from build123d import *

# Parameters (mm, degrees)
F0_R     = 0.4318
F1_DEPTH = 1.27


with BuildPart() as f1:
    # F0 (on Top) → F1 (new body)
    with BuildSketch(Plane.XY):
        with BuildLine():
            Line((12.65347, -2.153963), (4.316134, 2.261672))
            Line((4.316134, 2.261672), (4.327364, 12.763659))
            Line((4.327364, 12.763659), (4.156866, 12.998858))
            ThreePointArc((4.156866, 12.998858), (2.963087, 14.80923), (1.900066, 12.919114))
            Line((1.900066, 12.919114), (1.711051, 12.659542))
            Line((1.711051, 12.659542), (1.699981, 2.307537))
            Line((1.699981, 2.307537), (-5.691423, -1.091549))
            Line((-5.691423, -1.091549), (-5.691423, -2.478054))
            Line((-5.691423, -2.478054), (-5.310308, -2.303015))
            Line((-5.310308, -2.303015), (3.007935, 1.517402))
            Line((3.007935, 1.517402), (11.38347, -2.918464))
            Line((11.38347, -2.918464), (11.38347, -3.767079))
            Line((11.38347, -3.767079), (11.38347, -4.793607))
            Line((11.38347, -4.793607), (11.383473, -10.512839))
            Line((11.383473, -10.512839), (11.383474, -11.539368))
            Line((11.383474, -11.539368), (11.383474, -12.419249))
            Line((11.383474, -12.419249), (3.128473, -17.185279))
            Line((3.128473, -17.185279), (2.03357, -16.553137))
            Line((2.03357, -16.553137), (1.14457, -16.039872))
            Line((1.14457, -16.039872), (-3.808432, -13.180257))
            Line((-3.808432, -13.180257), (-5.529587, -12.419254))
            Line((-5.529587, -12.419254), (-5.691423, -3.510934))
            Line((-5.691423, -3.510934), (-6.522282, -3.510934))
            Line((-6.522282, -3.510934), (-6.580308, -3.439569))
            Line((-6.580308, -3.439569), (-6.396528, -9.918688))
            Line((-6.396528, -9.918688), (-16.026936, -16.915588))
            Line((-16.026936, -16.915588), (-16.107216, -17.162667))
            ThreePointArc((-16.107216, -17.162667), (-16.212667, -19.229532), (-14.225404, -18.651748))
            Line((-14.225404, -18.651748), (-13.96561, -18.651748))
            Line((-13.96561, -18.651748), (-6.396528, -13.152489))
            Line((-6.396528, -13.152489), (1.39857, -17.652989))
            Line((1.39857, -17.652989), (1.39857, -18.651748))
            Line((1.39857, -18.651748), (1.39857, -21.191748))
            Line((1.39857, -21.191748), (2.28757, -21.191748))
            Line((2.28757, -21.191748), (2.28757, -20.055981))
            Line((2.28757, -20.055981), (3.207054, -21.186821))
            Line((3.207054, -21.186821), (4.037913, -21.191748))
            Line((4.037913, -21.191748), (4.037913, -18.646821))
            Line((4.037913, -18.646821), (4.037913, -18.126682))
            Line((4.037913, -18.126682), (12.653472, -13.152485))
            Line((12.653472, -13.152485), (20.12443, -15.416135))
            Line((20.12443, -15.416135), (20.12443, -16.178135))
            Line((20.12443, -16.178135), (20.12443, -18.718135))
            Line((20.12443, -18.718135), (21.140028, -18.718135))
            Line((21.140028, -18.718135), (21.140028, -17.745525))
            Line((21.140028, -17.745525), (21.809838, -18.718135))
            Line((21.809838, -18.718135), (22.763277, -18.718135))
            Line((22.763277, -18.718135), (22.763277, -16.215688))
            Line((22.763277, -16.215688), (29.330721, -7.616372))
            Line((29.330721, -7.616372), (23.89467, 0.487487))
            Line((23.89467, 0.487487), (23.89467, 0.851521))
            Line((23.89467, 0.851521), (23.89467, 3.027487))
            Line((23.89467, 3.027487), (23.00567, 3.027487))
            Line((23.00567, 3.027487), (23.00567, 2.007953))
            Line((23.00567, 2.007953), (22.273508, 3.027487))
            Line((22.273508, 3.027487), (21.384508, 3.027487))
            Line((21.384508, 3.027487), (21.384508, 1.132124))
            Line((21.384508, 1.132124), (12.65347, -2.153963))
        make_face()
        with Locations((-15.424598, -18.233617)):
            Circle(F0_R, mode=Mode.SUBTRACT)
        with BuildLine():
            Line((-14.7405, -17.163612), (-6.396528, -11.017552))
            Line((-6.396528, -11.017552), (-6.396528, -12.053624))
            Line((-6.396528, -12.053624), (-14.247226, -17.75749))
            ThreePointArc((-14.247226, -17.75749), (-14.447644, -17.422161), (-14.7405, -17.163612))
        make_face(mode=Mode.SUBTRACT)
        Polygon((2.28757, -18.166253), (3.128473, -18.651748), (3.128473, -19.879702), (2.28757, -18.646821), align=None, mode=Mode.SUBTRACT)
        Polygon((21.874277, -17.244328), (21.140028, -16.178135), (21.140028, -15.723854), (21.874277, -15.946327), (21.874277, -16.178135), align=None, mode=Mode.SUBTRACT)
        Polygon((12.653474, -11.882485), (12.65347, -3.510934), (13.49167, -3.195462), (13.49167, -12.154831), align=None, mode=Mode.SUBTRACT)
        Polygon((27.564501, -6.689476), (28.079566, -7.398402), (22.323207, -15.02437), (21.47986, -14.75035), align=None, mode=Mode.SUBTRACT)
        Polygon((23.00567, 0.487487), (23.00567, -0.414785), (27.016591, -5.935343), (20.685605, -14.492281), (14.38067, -12.443685), (14.38067, -2.860871), (22.259525, 0.104481), (22.259525, 0.487487), (22.259525, 1.524642), align=None, mode=Mode.SUBTRACT)
        with BuildLine():
            Line((3.392922, 12.32978), (3.427035, 2.169838))
            Line((3.427035, 2.169838), (2.588835, 2.169838))
            Line((2.588835, 2.169838), (2.599707, 12.33742))
            ThreePointArc((2.599707, 12.33742), (2.995703, 12.270081), (3.392922, 12.32978))
        make_face(mode=Mode.SUBTRACT)
        with Locations((3.007935, 13.540022)):
            Circle(F0_R, mode=Mode.SUBTRACT)
        Polygon((-8.330766, -0.970934), (-7.652898, -0.970934), (-16.021372, 3.877039), (-16.676927, 2.740892), (-8.330766, -2.189404), align=None)
        Polygon((-5.691423, -2.478054), (-5.691423, -1.091549), (-5.691423, -0.970934), (-6.580423, -0.970934), (-6.580423, -2.198888), (-7.441766, -0.970934), (-7.652898, -0.970934), (-8.330766, -0.970934), (-8.330766, -2.189404), (-8.330766, -3.510934), (-7.441766, -3.510934), (-7.441766, -2.380094), (-6.580308, -3.439569), (-6.522282, -3.510934), (-5.691423, -3.510934), align=None)
        Polygon((24.531044, 11.272838), (23.00567, 3.027487), (23.89467, 3.027487), (23.89467, 0.851521), (25.779854, 11.04181), align=None)
    extrude(amount=F1_DEPTH)


solid = f1.part
Could you check a few things on this model? Use its own coordinates, in mm. A direction names the side the tool comes from. Give positions to 0.01 mm unless a question says otherwise; leave off trailing zeros. Write each loop counter-clockwise with the first axis right and the second up, starting at its lowest first coordinate (ties: lowest second). Pieces come first, ordered by that corner, then holes. Notation, with made-up numbers: (-16, 51) -> (-7, 51) arc R25 cw to (-7, 75) -> close; hole circle Ø10 at (75, 88.5). An arc over 180 degrees is marked (long way). Write each question's results on one line, items separated by ' | '. Start each with the question number.
Q1. I need wall thicknesses on probe 1 along Y at (x, z) = (-13, 0.1); probe 2 along X at (y, z) = (-6.5, 0.2); probe 3 along X at (y, z) = (-4, 0.45). Which ranges of each line are inside material? Lowest first, please.
Q2. I'm going to push flat-ended pins straight in: pin 1 Ø0.6 at (y, z) = (-7.5, 1) entering from -X; pin 2 Ø0.6 at (y, z) = (-2.5, 0.5) entering from +X; pin 3 Ø0.5 at (y, z) = (-11.5, 0.5) entering from -X. Where does each tip first touch, or does it pass through?
Q3. Suppose I cut it at C-C, the plane x = -12. List the corners of the cut face in (y, z) for me (3 decimals), and give its area (3 significant figures).
Q4. Which directions (+Z, -Z, +X, -X, +Y, -Y) give clear straight access to the entire face, cutting with the end or side of a thin tool? Please do faces 1 (the face through (20.124, -17, 1)), 2 (the face through (-6, -0.971, 1)), 3 (the face through (-8, -3.511, 1)), 4 (the face through (23.9, -10.15, 0.63)).
Q5. Suppose I cut it at A-A, the plane x = 16. List the corners of the cut face in (y, z) for me, and give its area (3 significant figures).
Q6. Suppose I cut it at D-D, the plane z = 0.35. State how many separate pieces and enclosed holes the cut face has, and give its area (3 significant figures).
Q7. Suppose I cut it at B-B, the plane y = -9. List the corners of the cut face in (x, z) for me, and give its area (3 significant figures).
Outcome:
1) probe 1: -17.95 to -16.85, -15.88 to -14.72, 0.57 to 2.13 | probe 2: -6.49 to -5.64, 11.38 to 12.65, 13.49 to 14.38, 26.6 to 28.58 | probe 3: -6.56 to -5.68, 11.38 to 12.65, 13.49 to 14.38, 25.61 to 26.9
2) pin 1: x = -6.47 | pin 2: x = 26.1 | pin 3: x = -8.92
3) outline: (-17.224, 0) -> (-16.125, 0) -> (-16.125, 1.27) -> (-17.224, 1.27) -> close; (-15.145, 0) -> (-13.99, 0) -> (-13.99, 1.27) -> (-15.145, 1.27) -> close; (-0.022, 0) -> (1.547, 0) -> (1.547, 1.27) -> (-0.022, 1.27) -> close | area: 4.86 mm2
4) face 1: +Z, -Z, -Y | face 2: +Z, -Z, +Y | face 3: +Z, -Z, -X | face 4: +Z, -Z
5) outline: (-14.17, 0) -> (-12.97, 0) -> (-12.97, 1.27) -> (-14.17, 1.27) -> close; (-2.25, 0) -> (-0.89, 0) -> (-0.89, 1.27) -> (-2.25, 1.27) -> close | area: 3.24 mm2
6) separate pieces: 1 | enclosed holes: 10 | area: 228 mm2
7) outline: (-6.42, 0) -> (-5.59, 0) -> (-5.59, 1.27) -> (-6.42, 1.27) -> close; (11.38, 0) -> (12.65, 0) -> (12.65, 1.27) -> (11.38, 1.27) -> close; (13.49, 0) -> (14.38, 0) -> (14.38, 1.27) -> (13.49, 1.27) -> close; (24.75, 0) -> (25.82, 0) -> (25.82, 1.27) -> (24.75, 1.27) -> close; (26.87, 0) -> (28.27, 0) -> (28.27, 1.27) -> (26.87, 1.27) -> close | area: 6.94 mm2
